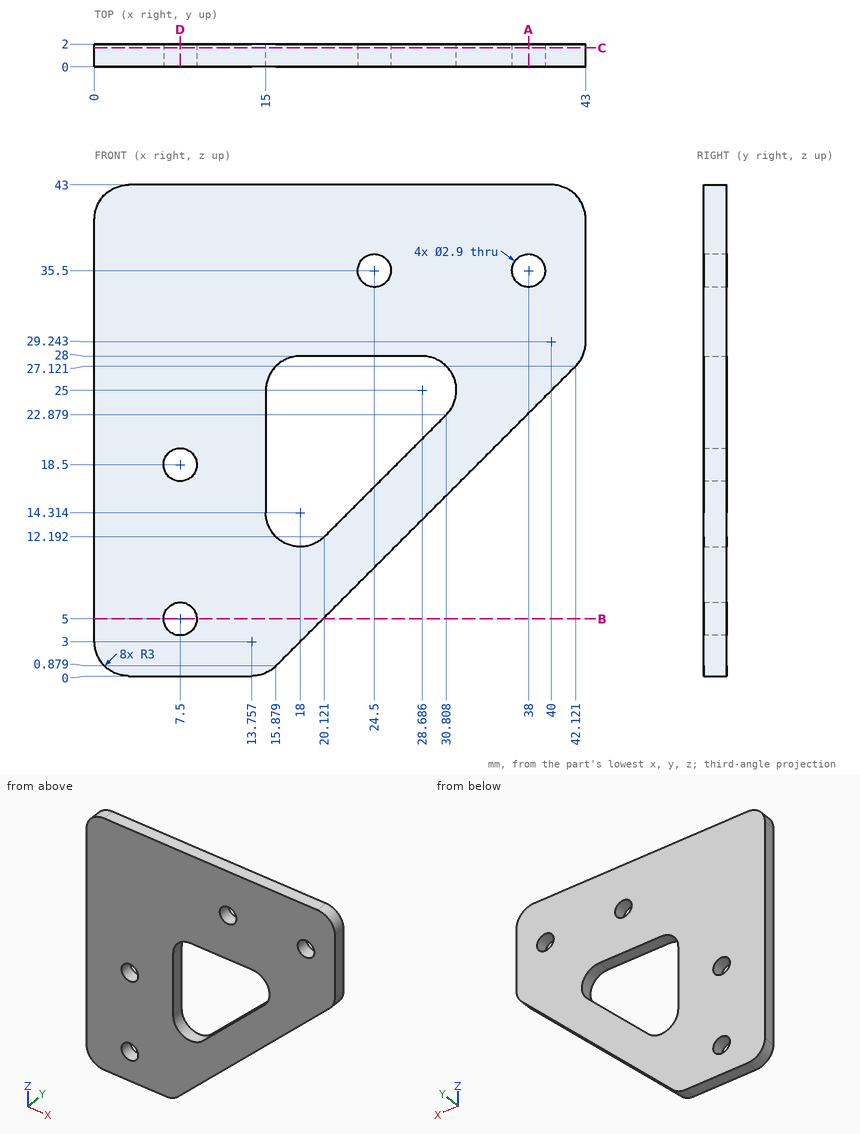
The figure shows three views and two pictorial views of one solid part (mm, origin at its lowest corner). Answer the questions. Round coordinates to 2 decimals unless told otherwise and drop trailing zeros. Write each loop counter-clockwise with the first axis right and the second up, starting at its lowest first coordinate (ties: lowest second). Pieces come first, ordered by that corner, then holes. Notation, with made-up numbers: (56.5, 52.25) - (70.5, 52.25) arc R22 ccw to (70.5, 85.25) - close; hole circle Ø10 at (-20.75, 9.5). An arc over 180 degrees is marked (long way). Answer in a Markdown table with one row per item. Add a question column.
1. A cutting plane is placed at A-A, the plane x = 38. Determine the outline of the cut face in (y, z), and give its area (3 significant figures).
2. Given pin 1 (0.6 mm diameter, centred on y = 1.5, z = 18.5, fed in from +X), flat-ended and moving along its own axis, determine where the tip first touches the part or whether it passes through.
3. A cutting plane is placed at C-C, the plane y = 1.65. Determine the outline of the cut face in (x, z), and give its area (3 significant figures).
4. A cutting plane is placed at B-B, the plane z = 5. Determine the outline of the cut face in (x, y), and give its area (3 significant figures).
5. A cutting plane is placed at D-D, the plane x = 7.5. Determine the outline of the cut face in (y, z).
6. Find the intervals of material crossed by line 1 along X through (y, z) = (1.5, 35.5); line 2 along X through (y, z) = (1.7, 25) (1 decimal); line 3 along X through (y, z) = (0.75, 18.5), in increasing order. Write a range as from..to.
Worked out:
| question | item | result |
|---|---|---|
| 1 | outline | (0, 23) - (2, 23) - (2, 34.05) - (0, 34.05) - close; (0, 36.95) - (2, 36.95) - (2, 43) - (0, 43) - close |
| 1 | area | 34.2 mm^2 |
| 2 | pin 1 | x = 33.8 |
| 3 | outline | (0, 3) arc R3 ccw to (3, 0) - (13.76, 0) arc R3 ccw to (15.88, 0.88) - (42.12, 27.12) arc R3 ccw to (43, 29.24) - (43, 40) arc R3 ccw to (40, 43) - (3, 43) arc R3 ccw to (0, 40) - close; hole circle Ø2.9 at (7.5, 5); hole circle Ø2.9 at (7.5, 18.5); hole (15, 14.31) arc R3 ccw to (20.12, 12.19) - (30.81, 22.88) arc R3 ccw to (28.69, 28) - (18, 28) arc R3 ccw to (15, 25) - close; hole circle Ø2.9 at (24.5, 35.5); hole circle Ø2.9 at (38, 35.5) |
| 3 | area | 1,230 mm^2 |
| 4 | outline | (0, 0) - (6.05, 0) - (6.05, 2) - (0, 2) - close; (8.95, 0) - (20, 0) - (20, 2) - (8.95, 2) - close |
| 4 | area | 34.2 mm^2 |
| 5 | outline | (0, 0) - (2, 0) - (2, 3.55) - (0, 3.55) - close; (0, 6.45) - (2, 6.45) - (2, 17.05) - (0, 17.05) - close; (0, 19.95) - (2, 19.95) - (2, 43) - (0, 43) - close |
| 6 | line 1 | 0..23.05, 25.95..36.55, 39.45..43 |
| 6 | line 2 | 0..15, 31.7..40 |
| 6 | line 3 | 0..6.05, 8.95..15, 26.43..33.5 |
